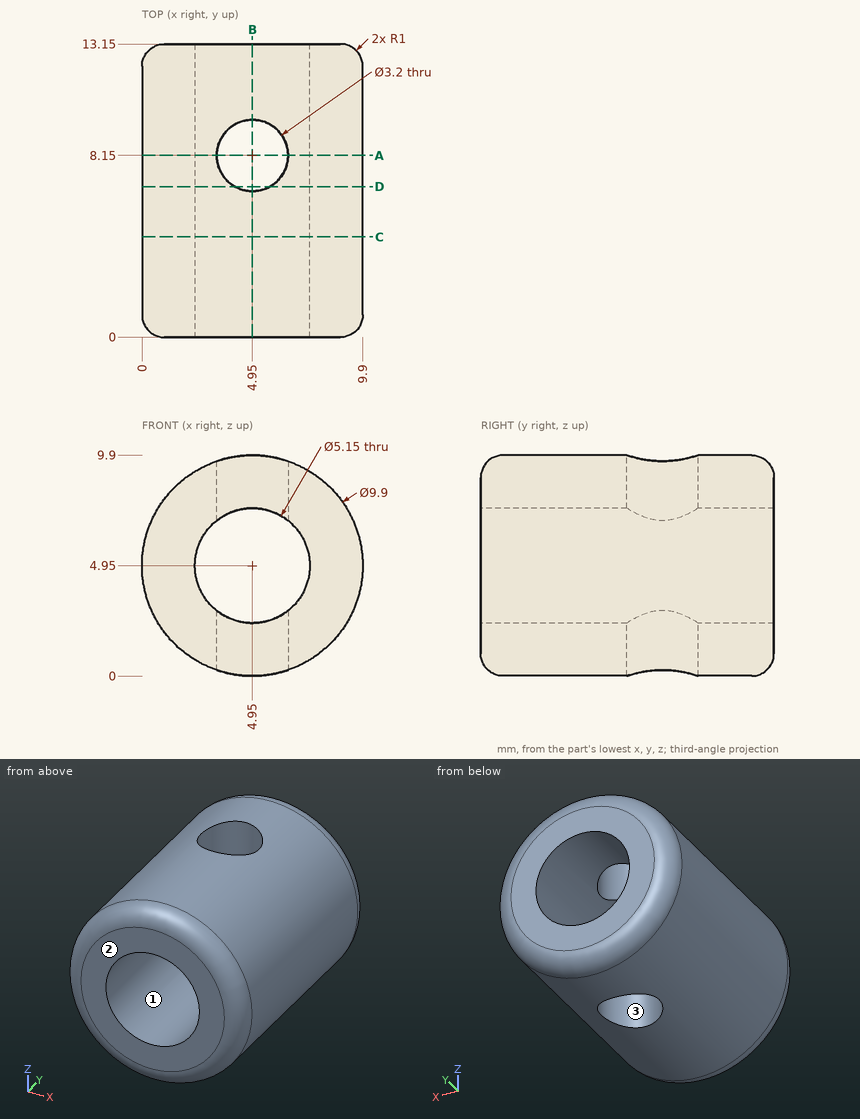
Geometry check sheet. Reference: drawing and pictorial views, mm from the part's lowest x, y, z. Round coordinates to 2 decimals unless told otherwise and drop trailing zeros. Loops run counter-clockwise (first coordinate to the right, second up) from the corner with the lowest first, then second, coordinate; pieces in that order, holes last. Notation, with made-up numbers: M 55.5,15.5 L 72.5,15.5 A27 cw 72.5,41.5 Z; hole C 9,-8.75 d6. An arc over 180 degrees is marked long. One line per item, written item: value.
(1) Sectioned sample at B-B, the plane x = 4.95. Count the separate pieces of the cut face and the enclosed holes in it, then the cut area to 3 significant figures.
Computed values:
separate pieces: 4
enclosed holes: 0
area: 46.4 mm^2
(2) Release check for a two-part mould opening along Y. For the marked faces 1, 2 and 3 record: +Y half, -Y half, draft (parallel to the pull), parting line (faces both ways), or undercut.
Computed values:
face 1: draft
face 2: -Y half
face 3: undercut
(3) Sectioned sample at C-C, the plane y = 4.5. Record the cut outline in (x, z) (3 decimals), then the cut area to 3 significant figures.
Computed values:
outline: C 4.95,4.95 d9.9; hole C 4.95,4.95 d5.15
area: 56.1 mm^2
(4) Depth check by flat-ended pin: pin 1 Ø3 at (x, z) = (4.95, 4.95) entering from -Y; pin 2 Ø2 at (y, z) = (5, 2.5) entering from +X; pin 3 Ø3 at (x, y) = (2.5, 9) entering from -Z; pin 4 Ø2 at (x, y) = (2.5, 4) entering from -Z. Enter the tip coordinate at first touch or a pass-through.
Computed values:
pin 1: passes through
pin 2: stops at x = 9.68
pin 3: stops at z = 0.1
pin 4: stops at z = 0.22
(5) Sectioned sample at A-A, the plane y = 8.15. Record the cut outline in (x, z) (3 decimals), then the cut area to 3 significant figures.
Computed values:
outline: M 3.35,0.266 L 3.35,2.932 A2.575 cw 3.35,6.968 L 3.35,9.634 A4.95 ccw Z; M 6.55,0.266 A4.95 ccw 6.55,9.634 L 6.55,6.968 A2.575 cw 6.55,2.932 Z
area: 40.4 mm^2
(6) Thickness scan on line 1 (Z direction, x = 4.95, y = 4) (3 decimals); line 2 (Y direction, x = 4.95, z = 8.75); line 3 (Z direction, x = 4, y = 10). Record the ranges inside material, lowest first.
Computed values:
line 1: z = 0 to 2.375, 7.525 to 9.9
line 2: y = 0 to 6.55, 9.75 to 13.15
line 3: z = 0.09 to 2.56, 7.34 to 9.81
(7) Sectioned sample at D-D, the plane y = 6.75. Record the cut outline in (x, z) (3 decimals), then the cut area to 3 significant figures.
Computed values:
outline: M 4.175,0.061 L 4.175,2.494 A2.575 cw 4.175,7.406 L 4.175,9.839 A4.95 ccw Z; M 5.725,0.061 A4.95 ccw 5.725,9.839 L 5.725,7.406 A2.575 cw 5.725,2.494 Z
area: 48.7 mm^2
